The listing builds one solid part. Answer for the finished solid, in the listing's coordinates (mm). Face numbers are marked on the shaded views. A direction names the side the tool comes from. Give positions to 0.01 mm unless a question says otherwise; leave off trailing zeros. Order: outer loops, then holes, each group sorted by start corner. A loop starts at its lowest first (then second) coordinate and runs counter-clockwise, first axis right, second up. Notation, with made-up numbers: M 75,39.25 L 116,39.25 A17 cw 116,54.25 Z; hole C 78.25,50.5 d8. An arc over 180 degrees is marked long. Answer as a JSON object with one key per item and string values. Group by question number.
```python
from build123d import *

# Parameters (mm, degrees)
CROQUIS2_W                 = 15
CROQUIS2_H                 = 15
SALIENTE_EXTRUIR1_DEPTH    = 4.5
CROQUIS3_W                 = 15
CROQUIS3_H                 = 10
CORTAR_EXTRUIR1_DEPTH      = 1.5
CORTAR_EXTRUIR2_DEPTH      = 12.521718622
CROQUIS10_W                = 4.5
CROQUIS10_H                = 9
SALIENTE_EXTRUIR4_DEPTH    = 10
CORTAR_EXTRUIR3_DEPTH      = 20.563997547
CORTAR_EXTRUIR3_DEPTH_BACK = 20.563997547
CROQUIS7_R                 = 1.5
REDONDEO2_R                = 1


with BuildPart() as part:
    # Croquis2 → Saliente-Extruir1 (new, symmetric)
    with BuildSketch(Plane.XY):
        Rectangle(CROQUIS2_W, CROQUIS2_H)
    extrude(amount=SALIENTE_EXTRUIR1_DEPTH, both=True)

    # Croquis3 → Cortar-Extruir1 (cut, symmetric)
    with BuildSketch(Plane.XY):
        with Locations((0, -2.5)):
            Rectangle(CROQUIS3_W, CROQUIS3_H)
    extrude(amount=CORTAR_EXTRUIR1_DEPTH, both=True, mode=Mode.SUBTRACT)

    # Croquis4 → Cortar-Extruir2 (cut, through all)
    with BuildSketch(Plane.XY):
        with BuildLine():
            Line((-1.5, 0), (-1.5, -7.5))
            Line((-1.5, -7.5), (1.5, -7.5))
            Line((1.5, -7.5), (1.5, 0))
            ThreePointArc((1.5, 0), (0, 1.5), (-1.5, 0))
        make_face()
    extrude(amount=-CORTAR_EXTRUIR2_DEPTH, mode=Mode.SUBTRACT)

    # Croquis10 → Saliente-Extruir4 (add)
    with BuildSketch(Plane(origin=(0, 7.5, 0), x_dir=(1, 0, 0), z_dir=(0, 1, 0))):
        with Locations((-5.25, 0)):
            Rectangle(CROQUIS10_W, CROQUIS10_H)
        with Locations((5.25, 0)):
            Rectangle(CROQUIS10_W, CROQUIS10_H)
    extrude(amount=SALIENTE_EXTRUIR4_DEPTH)

    # Croquis7 → Cortar-Extruir3 (cut, two sides: drawn at the far end of the back side and taken through both)
    with BuildSketch(Plane(origin=(0, 0, 0), x_dir=(0, 0, -1), z_dir=(1, 0, 0)).offset(-CORTAR_EXTRUIR3_DEPTH_BACK)):
        with Locations((0, 13.5)):
            Circle(CROQUIS7_R)
    extrude(amount=CORTAR_EXTRUIR3_DEPTH + CORTAR_EXTRUIR3_DEPTH_BACK, mode=Mode.SUBTRACT)

    # Redondeo2
    redondeo2_edges = [part.edges().sort_by_distance(p)[0] for p in [
        (5.25, 17.5, -4.5),
        (5.25, 17.5, 4.5),
        (-5.25, 17.5, 4.5),
        (-5.25, 17.5, -4.5),
    ]]
    fillet(redondeo2_edges, radius=REDONDEO2_R)


solid = part.part
```
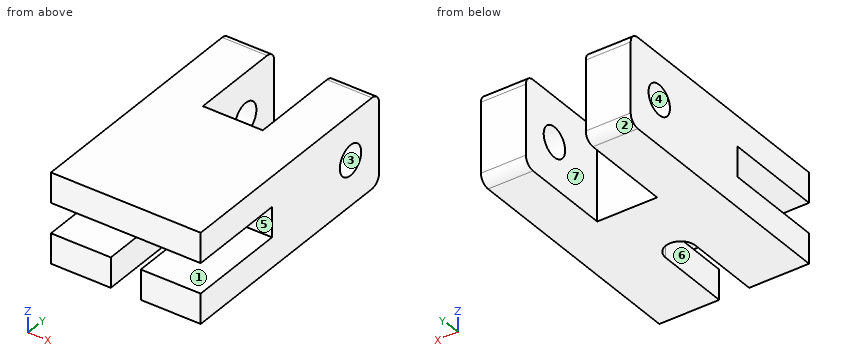
Item 1: Section D-D (y = -5.75) is taken. Determine the outline of the cut face in (x, z), and give its area (3 significant figures).
Item 2: Flat-ended cylindrical pins translate along their axes: P1, Ø0.9, axis at x = -0.5, z = 0.5, coming from the -Y side; P2, Ø1.8, axis at y = 13.5, z = 0, coming from the -X side. Find the tip coordinate at first contact, or state that the pin passes through.
Item 3: Section A-A (x = -5) is taken. Determine the outline of the cut face in (y, z), and give its area (3 significant figures).
Item 4: Consider probe 1 along X at (y, z) = (11.5, 4.25); probe 2 along Y at (x, z) = (4.6, 0); probe 3 along Z at (x, y) = (6, 13.5). Determine where each line is inside the solid, lowest interval first. Write a range as from..to.
Item 5: Determine the mould class of the marked faces 1, 2, 3 and 4 for opening direction Y: released by +Y, released by -Y, zero draft, split by the parting line, or undercut.
Item 6: Section C-C (y = 13.5) is taken. Determine the outline of the cut face in (x, z).
Item 7: A tool of negligible diameter and unlimited length cuts with its end or side. For the marked faces 5, 6 and 7, from which of +Z, -Z, +X, -X, +Y, -Y can it reach the whole face along a straight path? Write none if from no direction.
Item 8: Section B-B (z = 0) is taken. Determine the outline of the cut face in (x, y).
Values found:
{
 "1": {"outline": "M -7.5,-4.5 L -1.5,-4.5 L -1.5,-1.5 L -7.5,-1.5 Z; M -7.5,1.5 L 7.5,1.5 L 7.5,4.5 L -7.5,4.5 Z; M 1.5,-4.5 L 7.5,-4.5 L 7.5,-1.5 L 1.5,-1.5 Z", "area": "81.0 mm^2"},
 "2": {"P1": "stops at y = 2.5", "P2": "passes through"},
 "3": {"outline": "M -7.5,-4.5 L 16.5,-4.5 A1 ccw 17.5,-3.5 L 17.5,3.5 A1 ccw 16.5,4.5 L -7.5,4.5 L -7.5,1.5 L 2.5,1.5 L 2.5,-1.5 L -7.5,-1.5 Z; hole C 13.5,0 d3", "area": "188 mm^2"},
 "4": {"probe 1": "x = -7.5..-3, 3..7.5", "probe 2": "y = 2.5..12, 15..17.5", "probe 3": "z = -4.5..-1.5, 1.5..4.5"},
 "5": {"face 1": "zero draft", "face 2": "released by +Y", "face 3": "undercut", "face 4": "undercut"},
 "6": {"outline": "M -7.5,-4.5 L -3,-4.5 L -3,-1.5 L -7.5,-1.5 Z; M -7.5,1.5 L -3,1.5 L -3,4.5 L -7.5,4.5 Z; M 3,-4.5 L 7.5,-4.5 L 7.5,-1.5 L 3,-1.5 Z; M 3,1.5 L 7.5,1.5 L 7.5,4.5 L 3,4.5 Z"},
 "7": {"face 5": "+X, -X, -Y", "face 6": "-Z, -Y", "face 7": "+Z, -Z, +Y"},
 "8": {"outline": "M -7.5,2.5 L 7.5,2.5 L 7.5,12 L 3,12 L 3,7.5 L -3,7.5 L -3,12 L -7.5,12 Z; M -7.5,15 L -3,15 L -3,17.5 L -7.5,17.5 Z; M 3,15 L 7.5,15 L 7.5,17.5 L 3,17.5 Z"}
}
